Autodesk Inventor part; units mm, degrees
ref_plane "YZ Plane" through (0, 0, 0) normal (1, 0, 0) x (0, 1, 0)
ref_plane "XZ Plane" through (0, 0, 0) normal (0, 1, 0) x (-1, 0, 0)
ref_plane "XY Plane" through (0, 0, 0) normal (0, 0, 1) x (1, 0, 0)
sketch "Sketch1" plane through (0, 0, 0) normal (0, 0, 1) x (1, 0, 0)
  circle A0 centre (0, 0) radius 49
  dimension "d0" = 98
extrude "Extrusion1" add sketch "Sketch1" along normal blind 15
sketch "Sketch2" plane through (0, 0, 15) normal (0, 0, 1) x (1, 0, 0)
  circle A0 centre (0, 0) radius 35
  circle A1 centre (0, 35) radius 5
  circle A2 centre (-30.3109, 17.5) radius 5
  circle A3 centre (-30.3109, -17.5) radius 5
  circle A4 centre (0, -35) radius 5
  circle A5 centre (30.3109, -17.5) radius 5
  circle A6 centre (30.3109, 17.5) radius 5
  dimension "d3" = 70
  dimension "d4" = 10
  dimension "d7" = 360
extrude "Extrusion2" cut sketch "Sketch2" against normal up to next contours A6 A0 | A0 A6 | A5 A0 | A0 A5 | A1 A0 | A0 A1 | A4 A0 | A0 A4 | A2 A0 | A0 A2 | A3 A0 | A0 A3
sketch "Sketch3" plane through (0, 0, 15) normal (0, 0, 1) x (1, 0, 0)
  circle A0 centre (0, 0) radius 25
  dimension "d11" = 50
extrude "Extrusion3" add sketch "Sketch3" along normal blind 75
sketch "Sketch4" plane through (0, 0, 15) normal (0, 0, 1) x (1, 0, 0)
  circle A0 centre (0, 0) radius 13
  dimension "d14" = 26
extrude "Extrusion4" cut sketch "Sketch4" along normal blind 45
sketch "Sketch5" plane through (0, 0, 90) normal (0, 0, 1) x (1, 0, 0)
  line L0 (0, 0) -> (0, 50)
  line L1 (0, 0) -> (0, -50)
  arc A0 (-14.6459, -46.76) -> (14.6459, -46.76) centre (0, -50) ccw
  arc A1 (14.6459, 46.76) -> (-14.6459, 46.76) centre (0, 50) ccw
  circle A2 centre (0, 0) radius 49
  circle A3 centre (0, 50) radius 6
  circle A4 centre (0, -50) radius 6
  line L2 (-15, -50) -> (-28.4697, -9.4591)
  line L3 (15, -50) -> (28.4697, -9.4591)
  line L4 (-14.6459, 53.24) -> (-28.6072, 9.035)
  line L5 (14.6459, 53.24) -> (28.6072, 9.035)
  arc A5 (-28.6072, 9.035) -> (-28.4697, -9.4591) centre (0, 0) ccw
  arc A6 (28.4697, -9.4591) -> (28.6072, 9.035) centre (0, 0) ccw
  point P0 (16.254, -46.2256)
  point P1 (16.9391, 45.979)
  point P2 (-16.9391, 45.979)
  point P3 (-16.254, -46.2256)
  dimension "d17" = 50
  dimension "d18" = 50
  dimension "d19" = 30
  dimension "d20" = 30
  dimension "d22" = 12
  dimension "d23" = 12
extrude "Extrusion5" add sketch "Sketch5" against normal blind 15 contours L1 A4 A2 L2 A5 L4 A3 L0 | L0 A3 A2 L5 A6 L3 A4 L1 | A2 A1 A3 | A2 A0 A4 | A2 L4 A1 | A1 L5 A2 | A2 L3 A0 | A0 L2 A2
sketch "Sketch6" plane through (0, 0, 90) normal (0, 0, 1) x (1, 0, 0)
  line L0 (15, -50) -> (28.4697, -9.4591)
  arc A0 (28.4697, -9.4591) -> (28.6072, 9.035) centre (0, 0) ccw
  line L1 (28.6072, 9.035) -> (14.6459, 53.24)
  arc A1 (14.6459, 53.24) -> (-14.6459, 53.24) centre (0, 50) ccw
  line L2 (-14.6459, 53.24) -> (-28.6072, 9.035)
  arc A2 (-28.6072, 9.035) -> (-28.4697, -9.4591) centre (0, 0) ccw
  line L3 (-28.4697, -9.4591) -> (-15, -50)
  arc A3 (-15, -50) -> (15, -50) centre (0, -50) ccw
  circle A4 centre (0, -50) radius 6
  circle A5 centre (0, 50) radius 6
  circle A6 centre (0, 0) radius 17.5
  dimension "d26" = 35
extrude "Extrusion6" cut sketch "Sketch6" against normal blind 30 contours A6
properties part number "PIEZA_3D_2EX"
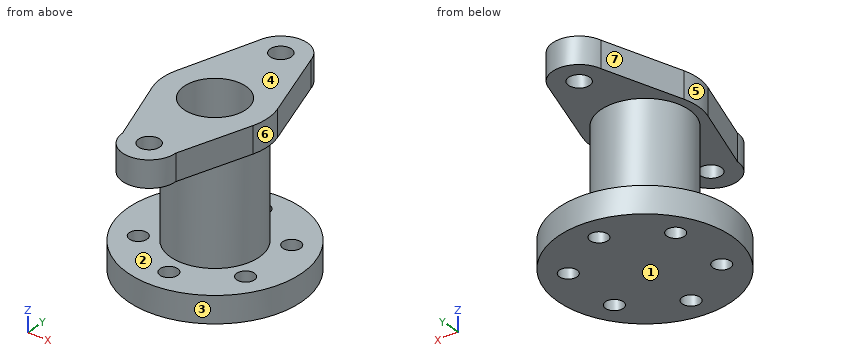
The listing builds one solid part. Answer for the finished solid, in the listing's coordinates (mm). Face numbers are marked on the shaded views. A direction names the side the tool comes from. Round coordinates to 2 decimals unless told otherwise and drop trailing zeros. Order: outer loops, then holes, each group sorted by start corner. A loop starts at its lowest first (then second) coordinate and runs counter-clockwise, first axis right, second up. Notation, with made-up numbers: (83.5, -37.5) -> (115.5, -37.5) arc R20 ccw to (115.5, -6.5) -> close; hole circle Ø6 at (-23, 62). An arc over 180 degrees is marked (long way). Put each result on its own line as item: value.
Q1. Section A-A, the plane y = 35 is taken. Write down the section's boundary in (x, z), and give its area (3 significant figures).
Results list:
outline: (-34.29, 0) -> (-5, 0) -> (-5, 15) -> (-34.29, 15) -> close; (-20.41, 75) -> (20.41, 75) -> (20.41, 90) -> (-20.41, 90) -> close; (5, 0) -> (34.29, 0) -> (34.29, 15) -> (5, 15) -> close
area: 1,490 mm^2
Q2. Which of the six approach directions +Z, -Z, +X, -X, +Y, -Y give full straight-line access (tool end or side, diameter ignored) to the marked faces 5, 6 and 7?
Results list:
face 5: +Z, -X
face 6: +Z, +X
face 7: +Z, -X, +Y
Q3. Section C-C, the plane y = -1.5 is taken. Write down the section's boundary in (x, z).
Results list:
outline: (-48.98, 0) -> (48.98, 0) -> (48.98, 15) -> (24.95, 15) -> (24.95, 75) -> (29.96, 75) -> (29.96, 90) -> (17.44, 90) -> (17.44, 60) -> (12.91, 60) -> (12.91, 15) -> (-12.91, 15) -> (-12.91, 60) -> (-17.44, 60) -> (-17.44, 90) -> (-29.96, 90) -> (-29.96, 75) -> (-24.95, 75) -> (-24.95, 15) -> (-48.98, 15) -> close
Q4. Each of these flat-tipped pins is pushed along its axis until it touches: P1, Ø9, axis at x = -30.31, y = 17.5, coming from the -Z side; P2, Ø8, axis at y = 5, z = 32.5, coming from the -X side; P3, Ø8, axis at x = 30.31, y = -17.5, coming from the +Z side; P4, Ø8, axis at x = 2, y = -2, coming from the +Z side. Where does it stop, or does it pass through?
Results list:
P1: z = 75
P2: x = -24.98
P3: through
P4: z = 15
Q5. Determine the mould class of the marked faces 1, 2, 3 and 4 for opening direction Z: pulls with the +Z half, pulls with the -Z half, needs draft (parallel to the pull), parting line crosses it, or undercut.
Results list:
face 1: pulls with the -Z half
face 2: undercut
face 3: needs draft
face 4: pulls with the +Z half
Q6. Section B-B, the plane z = 30.5 is taken. Write down the section's boundary in (x, y), and give its area (3 significant figures).
Results list:
outline: circle Ø50 at (0, 0); hole circle Ø26 at (0, 0)
area: 1,430 mm^2
Q7. Section D-D, the plane y = -32 is taken. Write down the section's boundary in (x, z), and give its area (3 significant figures).
Results list:
outline: (-37.11, 0) -> (-4, 0) -> (-4, 15) -> (-37.11, 15) -> close; (-20.98, 75) -> (20.98, 75) -> (20.98, 90) -> (-20.98, 90) -> close; (4, 0) -> (37.11, 0) -> (37.11, 15) -> (4, 15) -> close
area: 1,620 mm^2
Q8. Consider line 1 along Y through (x, z) = (0, 85.25); line 2 along Y through (x, z) = (-26, 8.5); line 3 along Z through (x, y) = (-28, -5.5). Determine where each line is inside the solid, lowest interval first.
Results list:
line 1: -65 to -56, -44 to -17.5, 17.5 to 44, 56 to 65
line 2: -41.53 to -20.03, -14.97 to 14.97, 20.03 to 41.53
line 3: 0 to 15, 75 to 90
